Verification items for the finished model (mm, model axes). Face numbers are marked on the shaded views. A direction names the side the tool comes from. Coordinates: 2 decimals unless noted, no trailing zeros. Loops run counter-clockwise (first coordinate to the right, second up) from the corner with the lowest first, then second, coordinate; pieces in that order, holes last.
Q1. Material ranges on probe 1 along Y at (x, z) = (0, 35.5); probe 2 along X at (y, z) = (-2, 17), recorded low to high.
Q2. Sectioned sample at A-A (z = 35). Enter the section's corners in (x, y), then the cut area to 3 significant figures.
Q3. Go/stop test with flat-tipped pins: P1, Ø4, axis at x = -2.5, z = 52.5, coming from the -Y side; P2, Ø2, axis at x = -3, y = 0.5, coming from the +Z side; P3, Ø5, axis at x = 0, z = 57, coming from the +Y side. Record where each tip stops, or that it passes through.
Q4. Access from +Z, -Z, +X, -X, +Y, -Y to the whole of each face (thin tool, end or side, straight path). Record for the marked faces 1 and 2.
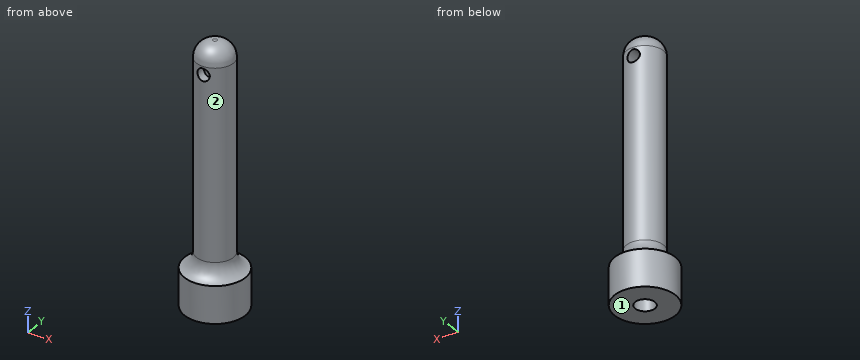
```python
from build123d import *

# Parameters (mm, degrees)
F0_R      = 7.4
F0_R_2    = 2.4
F1_DEPTH  = 3
F2_R      = 7.4
F3_DEPTH  = 3
F4_R      = 4.5
F4_R_2    = 2.4
F5_DEPTH  = 51
F6_DEPTH  = 3
F7_R      = 4.5
F8_DEPTH  = 6
F10_R     = 1.5
F11_DEPTH = 12.5


# Not quite as in the source:
# - a fillet or chamfer that OpenCascade refuses, or shapes differently, is made with other operations: its cross-section is extruded or revolved along the edge and cut away or added


with BuildPart() as f1:
    # F0 (on Top) → F1 (new body)
    with BuildSketch(Plane.XY):
        Circle(F0_R)
        Circle(F0_R_2, mode=Mode.SUBTRACT)
    extrude(amount=F1_DEPTH)

    # F2 (on face) → F3 (join)
    with BuildSketch(Plane.XY.offset(3)):
        Circle(F2_R)
        Polygon((0, 4.1569219382), (3.6, 2.0784609691), (3.6, -2.0784609691), (0, -4.1569219382), (-3.6, -2.0784609691), (-3.6, 2.0784609691), align=None, mode=Mode.SUBTRACT)
    extrude(amount=F3_DEPTH)

    # F4 (on face) → F5 (join)
    with BuildSketch(Plane.XY.offset(6)):
        Circle(F4_R)
        Polygon((-3.6, -2.0784609691), (-3.6, 2.0784609691), (0, 4.1569219382), (3.6, 2.0784609691), (3.6, -2.0784609691), (0, -4.1569219382), align=None, mode=Mode.SUBTRACT)
        Polygon((0, 4.1569219382), (-3.6, 2.0784609691), (-3.6, -2.0784609691), (0, -4.1569219382), (3.6, -2.0784609691), (3.6, 2.0784609691), align=None)
        Circle(F4_R_2, mode=Mode.SUBTRACT)
    extrude(amount=F5_DEPTH)

    # F6 (add): a face of the model
    f6_faces = [f1.faces().sort_by_distance(p)[0] for p in [
        (-7.1906963928, 0, 6),
    ]]
    extrude(f6_faces, amount=F6_DEPTH)

    # F7 (on face) → F8 (join)
    with BuildSketch(Plane.XY.offset(57)):
        Circle(F7_R)
    extrude(amount=F8_DEPTH)

    # F9: fillet of radius 4 on 2 edges, made by hand

    # F9_s1 → F9_t2 (revolve)
    with BuildSketch(Plane.XZ):
        with BuildLine():
            ThreePointArc((7.4, 9), (5.3062561155, 10.4374579888), (4.5, 12.8457769046))
            Line((4.5, 12.8457769046), (4.5, 9))
            Line((4.5, 9), (7.4, 9))
        make_face()
    revolve(axis=Axis((0, 0, 9), (0, 0, 1)))

    # F9_s3 → F9_t4 (revolve, cut)
    with BuildSketch(Plane.XZ):
        with BuildLine():
            ThreePointArc((4.5, 59), (3.3284271247, 61.8284271247), (0.5, 63))
            Line((0.5, 63), (4.5, 63))
            Line((4.5, 63), (4.5, 59))
        make_face()
    revolve(axis=Axis((0, 0, 63), (0, 0, 1)), mode=Mode.SUBTRACT)

    # F10 (on Front) → F11 (cut, symmetric)
    with BuildSketch(Plane.XZ):
        with Locations((0, 57)):
            Circle(F10_R)
    extrude(amount=F11_DEPTH, both=True, mode=Mode.SUBTRACT)


solid = f1.part
```
Geometry check:
1. probe 1: y = -4.5 to -2.4, 2.4 to 4.5
1. probe 2: x = -4.03 to -1.33, 1.33 to 4.03
2. outline: circle Ø9 at (0, 0); hole circle Ø4.8 at (0, 0)
2. area: 45.5 mm2
3. P1: stops at y = -4.47
3. P2: stops at z = 62.69
3. P3: stops at y = 4.5
4. face 1: -Z, +X, -X, +Y, -Y
4. face 2: +Z
